Autodesk Inventor part; units mm, degrees
ref_plane "YZ Plane" through (0, 0, 0) normal (1, 0, 0) x (0, 1, 0)
ref_plane "XZ Plane" through (0, 0, 0) normal (0, 1, 0) x (-1, 0, 0)
ref_plane "XY Plane" through (0, 0, 0) normal (0, 0, 1) x (1, 0, 0)
sketch "Sketch1" plane through (0, 0, 0) normal (1, 0, 0) x (0, 1, 0)
  line L0 (-12.4, 9) -> (10.6, 9)
  line L1 (10.6, 9) -> (10.6, -9)
  line L2 (10.6, -9) -> (-12.4, -9)
  line L3 (-12.4, -9) -> (-12.4, 9)
  circle A0 centre (7.55, 0) radius 0.9
  circle A1 centre (-9.35, 0) radius 0.9
  line L4 (-0.9, 9) -> (-0.9, -9) construction
  line L5 (8.45, 0) -> (-10.25, 0) construction
  point P0 (-0.9, 0)
  point P1 (-0.9, 0)
  dimension "d5" = 1.8
  dimension "d6" = 1.8
  dimension "d0" = 23
  dimension "d1" = 18
  dimension "d4" = 16.9
extrude "Extrusion1" add sketch "Sketch1" along normal blind 2
hole "Hole1" at (2, 7.55, 0) direction (-1, 0, 0) diameter 1.8 depth 15 tip angle 118 countersink diameter 4 countersink angle 90
hole "Hole2" at (2, -9.3379, 0.0682) direction (-1, 0, 0) diameter 1.8 depth 15 tip angle 118 countersink diameter 4 countersink angle 90
equation "\"d6\" = d5"
properties part number "USB-bay_cover"
Geometry: final body of the model. Coordinates: model frame, mm. Coordinates: 2 decimals unless noted, no trailing zeros. Order: outer loops, then holes, each group sorted by start corner. A loop starts at its lowest first (then second) coordinate and runs counter-clockwise, first axis right, second up.
1) Draft query along Z for faces 1 (the cylindrical face through (0.4, 8.4, -0.3)), 2 (the flat face through (1, -1, -9)), 3 (the flat face through (1, 10.6, 0)). Return one class per face: released by +Z, released by -Z, zero draft, split by the parting line, or undercut.
Result sheet:
face 1: undercut
face 2: released by -Z
face 3: zero draft
2) Section B-B (x = 1.55). Return loops of the section in (y, z), then the cut area to 3 significant figures.
Result sheet:
outline: (-12.4, -9) - (10.6, -9) - (10.6, 9) - (-12.4, 9) - close; hole circle Ø3.1 at (-9.34, 0.07); hole circle Ø3.1 at (7.55, 0)
area: 399 mm2
3) Ray query, probe 1 along Y at (x, z) = (0.2, 0); probe 2 along Z at (x, y) = (0.45, 7.55); probe 3 along Z at (x, y) = (0.8, -9). Return the intervals inside material, ascending.
Result sheet:
probe 1: y = -12.4 to -10.25, -8.44 to 6.65, 8.45 to 10.6
probe 2: z = -9 to -0.9, 0.9 to 9
probe 3: z = -9 to -0.83, 0.9 to 9
4) Section A-A (y = 7.55). Return loops of the section in (x, z).
Result sheet:
outline: (0, -9) - (2, -9) - (2, -2) - (0.9, -0.9) - (0, -0.9) - close; (0, 0.9) - (0.9, 0.9) - (2, 2) - (2, 9) - (0, 9) - close
